The model under review builds one solid part; all positions refer to its coordinate system, in mm. Coordinates: 2 decimals unless noted, no trailing zeros. Write each loop counter-clockwise with the first axis right and the second up, starting at its lowest first coordinate (ties: lowest second). Pieces come first, ordered by that corner, then holes. Notation, with made-up numbers: (-23.75, 31.5) - (32.25, 31.5) arc R20 cw to (32.25, 47.5) - close; hole circle Ø2 at (30, -26). An arc over 180 degrees is marked (long way). Put each result on its own line as item: value. Start each with the question number.
Item 1: Consider section A-A on x = 1107. Give the boundary of the cut face in (y, z).
Item 2: Consider section B-B on z = 32. Give the boundary of the cut face in (x, y), then the cut area to 3 significant figures.
Item 3: To check wall thickness, follow L1, parallel to Z at x = 425.5, y = -2; L2, parallel to Y at x = 369.5, z = 31. State the ranges of each line that lie inside material, in increasing order. Write a range as [from, to].
```python
from build123d import *

# Parameters (mm, degrees)
F0_W     = 2032
F0_H     = 15
F1_DEPTH = 7.5
F2_W     = 5
F2_H     = 5
F3_DEPTH = 2032


with BuildPart() as f1:
    # F0 (on Front) → F1 (new body, symmetric)
    with BuildSketch(Plane.XZ):
        with Locations((966.749246, 32.093956)):
            Rectangle(F0_W, F0_H)
    extrude(amount=F1_DEPTH, both=True)

    # F2 (on face) → F3 (cut)
    with BuildSketch(Plane(origin=(-49.250754, 0, 0), x_dir=(0, -1, 0), z_dir=(-1, 0, 0))):
        with Locations((0, 32.093956)):
            Rectangle(F2_W, F2_H)
    extrude(amount=-F3_DEPTH, mode=Mode.SUBTRACT)


solid = f1.part
```
Report:
1. outline: (-7.5, 24.59) - (7.5, 24.59) - (7.5, 39.59) - (-7.5, 39.59) - close; hole (-2.5, 29.59) - (2.5, 29.59) - (2.5, 34.59) - (-2.5, 34.59) - close
2. outline: (-49.25, -7.5) - (1982.75, -7.5) - (1982.75, -2.5) - (-49.25, -2.5) - close; (-49.25, 2.5) - (1982.75, 2.5) - (1982.75, 7.5) - (-49.25, 7.5) - close
2. area: 20,300 mm²
3. L1: [24.59, 29.59], [34.59, 39.59]
3. L2: [-7.5, -2.5], [2.5, 7.5]
